Can you work these out from the model? Positions are in its coordinate system, mm. A direction names the side the tool comes from. Coordinates: 2 decimals unless noted, no trailing zeros. Loops run counter-clockwise (first coordinate to the right, second up) from the corner with the lowest first, then second, coordinate; pieces in that order, holes last.
Solid Edge part; units mm, degrees
sketch "Sketch1" plane through (0, 0, 0) normal (0, -1, 0) x (1, 0, 0)
  line L0 (-60, 4) -> (-38, 4)
  line L1 (-38, 4) -> (-38, 8)
  arc A0 (-38, 8) -> (-30, 0) centre (-38, 0) cw
  line L2 (-60, 4) -> (-60, 0)
revolve "RevolvedProtrusion1" add sketch "Sketch1" angle 360 about axis through (-60, 0, 0) along (1, 0, 0)
sketch "Sketch2" plane through (0, 0, 0) normal (0, -1, 0) x (1, 0, 0)
  line L0 (-33, -1) -> (-30, -1)
  line L1 (-30, -1) -> (-30, 1)
  line L2 (-30, 1) -> (-33, 1)
  line L3 (-33, 1) -> (-33, -1)
extrude "Cutout1" cut sketch "Sketch2" along normal mid plane 74.7625
cosmetic_thread "Thread1"
chamfer "Chamfer_1" distance 0.5 angle 45 1 edges at (-60, 0, -4)
Item 1: Suppose I cut it at C-C, the plane x = -42. Please give me the cut outline in (y, z).
Results are:
outline: circle Ø8 at (0, 0)
Item 2: On a 3-axis mill with a long thin cutter (end or side, diameter ignored), from which of +Z, -Z, +X, -X, +Y, -Y can I reach the whole of each face in a straight line? I mean faces 4 (the face through (-60, 0, 0)), 5 (the face through (-32, 0, 1)). Say none if no direction works.
Results are:
face 4: +Z, -Z, -X, +Y, -Y
face 5: +X, +Y, -Y
Item 3: Suppose I cut it at B-B, the plane z = 0. Please give me the cut outline in (x, y) (3 decimals).
Results are:
outline: (-60, -3.5) - (-59.5, -4) - (-38, -4) - (-38, -8) arc R8 ccw to (-33, -6.245) - (-33, 6.245) arc R8 ccw to (-38, 8) - (-38, 4) - (-59.5, 4) - (-60, 3.5) - close
Item 4: I need wall thicknesses on line 1 along X through (y, z) = (-2.75, 0.75); line 2 along Z through (x, y) = (-37.25, 1.75); line 3 along X through (y, z) = (-3.5, 5). Which ranges of each line are inside material? Lowest first, please.
Results are:
line 1: x = -60 to -33
line 2: z = -7.77 to 7.77
line 3: x = -38 to -32.83
Item 5: We'd pull the mould along Z, two halves only. Please class faces 1 (the face through (-32, 0, -1)), 2 (the face through (-38, 2, -4)), 3 (the face through (-48.6, 3.905, -0.867)): +Z half, -Z half, draft (parallel to the pull), parting line (faces both ways), or undercut.
Results are:
face 1: undercut
face 2: draft
face 3: parting line
Item 6: Suppose I cut it at D-D, the plane y = 5.75. Please give me the cut outline in (x, z).
Results are:
outline: (-38, -5.56) arc R5.56 ccw to (-32.53, -1) - (-33, -1) - (-33, 1) - (-32.53, 1) arc R5.56 ccw to (-38, 5.56) - close
Item 7: Suppose I cut it at A-A, the plane y = 0. Please give me the cut outline in (x, z), plus the area to 3 significant figures.
Results are:
outline: (-60, -3.5) - (-59.5, -4) - (-38, -4) - (-38, -8) arc R8 ccw to (-30.06, -1) - (-33, -1) - (-33, 1) - (-30.06, 1) arc R8 ccw to (-38, 8) - (-38, 4) - (-59.5, 4) - (-60, 3.5) - close
area: 270 mm2
Item 8: I'm going to push flat-ended pins straight in: P1, Ø3, axis at x = -56, z = -1, coming from the +Y side; P2, Ø3, axis at y = 4.5, z = 6, coming from the +X side; P3, Ø3, axis at x = -33.5, y = -2.5, coming from the -Z side. Where does each tip first touch, or does it pass through?
Results are:
P1: stops at y = 4
P2: stops at x = -32.71
P3: stops at z = -7.12
